Work out the finished part from the listing and answer in its coordinate system (mm). A direction names the side the tool comes from. Coordinates: 2 decimals unless noted, no trailing zeros. Loops run counter-clockwise (first coordinate to the right, second up) from the corner with the lowest first, then second, coordinate; pieces in that order, holes last. Notation, with made-up numbers: (60, 6.5) -> (115, 6.5) arc R25 ccw to (115, 36.5) -> close; hole circle Ø10 at (31, 6). An arc over 180 degrees is marked (long way). One line per question, with ' | ' between items.
```python
from build123d import *

# Parameters (mm, degrees)
BOSS_EXTRU_1_DEPTH      = 2
BOSS_EXTRU_2_DEPTH      = 4
ESQUISSE3_W             = 68
ESQUISSE3_H             = 60
ESQUISSE3_W_2           = 56
ESQUISSE3_H_2           = 48
BOSS_EXTRU_3_DEPTH      = 2
ESQUISSE4_W             = 60
ESQUISSE4_H             = 52
ESQUISSE4_W_2           = 56
ESQUISSE4_H_2           = 48
BOSS_EXTRU_4_DEPTH      = 13
ESQUISSE5_W             = 56
ESQUISSE5_H             = 48
BOSS_EXTRU_5_DEPTH      = 2
ESQUISSE6_W             = 20
ESQUISSE6_H             = 10
ENL_V_MAT_EXTRU_1_DEPTH = 35


with BuildPart() as part:
    # Esquisse1 → Boss.-Extru.1 (new body)
    with BuildSketch(Plane.XY):
        Polygon((-50, 68), (-50, -68), (-10, -68), (10, -68), (50, -68), (50, 68), align=None)
        Polygon((-10, 3), (-34, 3), (-34, 63), (34, 63), (34, 3), (10, 3), (10, -37), (-10, -37), align=None, mode=Mode.SUBTRACT)
    extrude(amount=BOSS_EXTRU_1_DEPTH)

    # Esquisse2 → Boss.-Extru.2 (add)
    with BuildSketch(Plane.XY.offset(2)):
        Polygon((36, 65), (-36, 65), (-36, 1), (-10, 1), (-10, 3), (-34, 3), (-34, 63), (34, 63), (34, 3), (10, 3), (10, 1), (36, 1), align=None)
    extrude(amount=BOSS_EXTRU_2_DEPTH)

    # Esquisse3 → Boss.-Extru.3 (add)
    with BuildSketch(Plane.XY.offset(6)):
        with Locations((0, 33)):
            Rectangle(ESQUISSE3_W, ESQUISSE3_H)
        with Locations((0, 33)):
            Rectangle(ESQUISSE3_W_2, ESQUISSE3_H_2, mode=Mode.SUBTRACT)
    extrude(amount=-BOSS_EXTRU_3_DEPTH)

    # Esquisse4 → Boss.-Extru.4 (add)
    with BuildSketch(Plane.XY.offset(6)):
        with Locations((0, 33)):
            Rectangle(ESQUISSE4_W, ESQUISSE4_H)
        with Locations((0, 33)):
            Rectangle(ESQUISSE4_W_2, ESQUISSE4_H_2, mode=Mode.SUBTRACT)
    extrude(amount=BOSS_EXTRU_4_DEPTH)

    # Esquisse5 → Boss.-Extru.5 (add)
    with BuildSketch(Plane.XY.offset(19)):
        with Locations((0, 33)):
            Rectangle(ESQUISSE5_W, ESQUISSE5_H)
    extrude(amount=-BOSS_EXTRU_5_DEPTH)

    # Esquisse6 → Enlèv. mat.-Extru.1 (cut)
    with BuildSketch(Plane.XY.offset(19)):
        with Locations((0, 6)):
            Rectangle(ESQUISSE6_W, ESQUISSE6_H)
    extrude(amount=-ENL_V_MAT_EXTRU_1_DEPTH, mode=Mode.SUBTRACT)


solid = part.part
```
1) Find section D-D (x = -26). Write down the section's boundary in (y, z), plus the area to 3 significant figures.
Check values:
outline: (-68, 0) -> (3, 0) -> (3, 4) -> (9, 4) -> (9, 17) -> (57, 17) -> (57, 4) -> (63, 4) -> (63, 0) -> (68, 0) -> (68, 2) -> (65, 2) -> (65, 6) -> (59, 6) -> (59, 19) -> (7, 19) -> (7, 6) -> (1, 6) -> (1, 2) -> (-68, 2) -> close | area: 340 mm^2
2) Flat-ended cylindrical pins translate along their axes: pin 1 (4.5 mm diameter, centred on x = 21.5, z = 4, fed in from -Y); pin 2 (6.5 mm diameter, centred on x = -11.5, z = 11.5, fed in from -Y); pin 3 (4 mm diameter, centred on x = -18, z = 12, fed in from +Y); pin 4 (4 mm diameter, centred on y = 24.5, z = 11.5, fed in from -X). Find the tip coordinate at first contact, or state that the pin passes through.
Check values:
pin 1: stops at y = -68 | pin 2: stops at y = 7 | pin 3: stops at y = 59 | pin 4: stops at x = -30
3) Find section B-B (x = -0.5). Write down the section's boundary in (y, z), plus the area to 3 significant figures.
Check values:
outline: (-68, 0) -> (-37, 0) -> (-37, 2) -> (-68, 2) -> close; (11, 17) -> (57, 17) -> (57, 4) -> (63, 4) -> (63, 0) -> (68, 0) -> (68, 2) -> (65, 2) -> (65, 6) -> (59, 6) -> (59, 19) -> (11, 19) -> close | area: 210 mm^2
4) Find the intervals of material crossed by line 1 along Y through (x, z) = (25, 11.5); line 2 along X through (y, z) = (25.5, 7.5); line 3 along X through (y, z) = (8, 13.5), in increasing order.
Check values:
line 1: y = 7 to 9, 57 to 59 | line 2: x = -30 to -28, 28 to 30 | line 3: x = -30 to -10, 10 to 30
5) For faces 4 (the face through (28, 33, 10)), 5 (the face through (23, 1, 4)), 6 (the face through (0, 59, 12)), determine the directions among +Z, -Z, +X, -X, +Y, -Y from which every point of the face is accessible in a straight line to the end or side of a thin tool.
Check values:
face 4: -Z | face 5: +Z, +X, -X, -Y | face 6: +Z, +X, -X, +Y
6) Find section C-C (z = 9.75). Write down the section's boundary in (x, y).
Check values:
outline: (-30, 7) -> (-10, 7) -> (-10, 9) -> (-28, 9) -> (-28, 57) -> (28, 57) -> (28, 9) -> (10, 9) -> (10, 7) -> (30, 7) -> (30, 59) -> (-30, 59) -> close
7) The mould has two halves that part along X. Classify faces 1 (the face through (36, 33, 4)), 2 (the face through (0, 63, 2)), 3 (the face through (0, 33, 19)): released by +X, released by -X, zero draft, split by the parting line, or undercut.
Check values:
face 1: released by +X | face 2: undercut | face 3: zero draft
8) Find section A-A (y = -33.5). Write down the section's boundary in (x, z), plus the area to 3 significant figures.
Check values:
outline: (-50, 0) -> (-10, 0) -> (-10, 2) -> (-50, 2) -> close; (10, 0) -> (50, 0) -> (50, 2) -> (10, 2) -> close | area: 160 mm^2
